```python
from build123d import *

# Parameters (mm, degrees)
BOSS_EXTRUDE1_DEPTH = 13.5
SKETCH2_W           = 45
SKETCH2_H           = 45
CUT_EXTRUDE1_DEPTH  = 11.72
SKETCH3_R           = 13.5
CUT_EXTRUDE2_DEPTH  = 84.329160712
CHAMFER1_SIZE       = 3
SKETCH7_W           = 113.25
SKETCH7_H           = 1.5
CUT_EXTRUDE4_DEPTH  = 84.598089841
CHAMFER2_SIZE       = 3
CHAMFER2_SIZE2      = 5.196152423
SKETCH8_R           = 2.25
CUT_EXTRUDE5_DEPTH  = 82.936336555
CUT_EXTRUDE6_START  = -4
SKETCH9_R           = 4.5
CUT_EXTRUDE6_DEPTH  = 78.936336555
SKETCH5_R           = 1.75
CUT_EXTRUDE7_DEPTH  = 84.013934059


with BuildPart() as part:
    # Sketch1 → Boss-Extrude1 (new body)
    with BuildSketch(Plane(origin=(0, 0, 0), x_dir=(1, 0, 0), z_dir=(0, 1, 0))):
        Polygon((-56.625, 0), (56.625, 0), (21.983983849, 60), (-21.983983849, 60), align=None)
    extrude(amount=BOSS_EXTRUDE1_DEPTH)

    # Sketch2 → Cut-Extrude1 (cut)
    with BuildSketch(Plane.XZ):
        with Locations((0, -31.45)):
            Rectangle(SKETCH2_W, SKETCH2_H)
    extrude(amount=-CUT_EXTRUDE1_DEPTH, mode=Mode.SUBTRACT)

    # Sketch3 → Cut-Extrude2 (cut, through all)
    with BuildSketch(Plane.XZ.offset(-11.72)):
        with Locations(Location((0, -31.45, 0), (0, 0, 270))):
            Circle(SKETCH3_R)
    extrude(amount=-CUT_EXTRUDE2_DEPTH, mode=Mode.SUBTRACT)

    # Chamfer1
    chamfer1_edges = [part.edges().sort_by_distance(p)[0] for p in [
        (-22.5, 5.86, -8.95),
        (-22.5, 5.86, -53.95),
        (22.5, 5.86, -53.95),
        (22.5, 5.86, -8.95),
    ]]
    chamfer(chamfer1_edges, length=CHAMFER1_SIZE)

    # Sketch7 → Cut-Extrude4 (cut, through all)
    with BuildSketch(Plane(origin=(0, 13.5, 0), x_dir=(1, 0, 0), z_dir=(0, 1, 0))):
        with Locations((0, 0.75)):
            Rectangle(SKETCH7_W, SKETCH7_H)
    extrude(amount=-CUT_EXTRUDE4_DEPTH, mode=Mode.SUBTRACT)

    # Chamfer2
    chamfer2_edges = [part.edges().sort_by_distance(p)[0] for p in [
        (0, 13.5, -1.5),
    ]]
    chamfer2_side = [part.faces().sort_by_distance(p)[0] for p in [
        (0, 6.75, -1.5),
    ]]
    chamfer(chamfer2_edges, length=CHAMFER2_SIZE, length2=CHAMFER2_SIZE2, reference=chamfer2_side[0])

    # Sketch8 → Cut-Extrude5 (cut, through all)
    with BuildSketch(Plane.XY.offset(-1.5)):
        with Locations((-40, 5)):
            Circle(SKETCH8_R)
        with Locations((40, 5)):
            Circle(SKETCH8_R)
    extrude(amount=-CUT_EXTRUDE5_DEPTH, mode=Mode.SUBTRACT)

    # Sketch9 → Cut-Extrude6 (cut, through all)
    with BuildSketch(Plane.XY.offset(-1.5).offset(CUT_EXTRUDE6_START)):
        with Locations((-40, 5)):
            Circle(SKETCH9_R)
        with Locations((40, 5)):
            Circle(SKETCH9_R)
    extrude(amount=-CUT_EXTRUDE6_DEPTH, mode=Mode.SUBTRACT)

    # Sketch5 → Cut-Extrude7 (cut, through all)
    with BuildSketch(Plane(origin=(0, 13.5, 0), x_dir=(1, 0, 0), z_dir=(0, 1, 0))):
        with Locations(Location((15.5, 46.95, 0), (0, 0, 270))):
            Circle(SKETCH5_R)
        with Locations(Location((15.5, 15.95, 0), (0, 0, 270))):
            Circle(SKETCH5_R)
        with Locations(Location((-15.5, 15.95, 0), (0, 0, 270))):
            Circle(SKETCH5_R)
        with Locations(Location((-15.5, 46.95, 0), (0, 0, 270))):
            Circle(SKETCH5_R)
    extrude(amount=-CUT_EXTRUDE7_DEPTH, mode=Mode.SUBTRACT)


solid = part.part
```
CAD build for the part. Positions are in the model's coordinates, mm. A direction names the side the tool comes from. Coordinates: 2 decimals unless noted, no trailing zeros. Order: outer loops, then holes, each group sorted by start corner. A loop starts at its lowest first (then second) coordinate and runs counter-clockwise, first axis right, second up.
(1) Which spindle directions (+Z, -Z, +X, -X, +Y, -Y) get a long thin tool onto all of the face, cutting with end or side? Do faces 4 (the face through (-38, 3, -5.5)), 5 (the face through (-20.98, 5.78, -10.43)), 6 (the face through (37.752, 5.099, -3.472)). Say none if no direction does.
Solution:
face 4: -Z
face 5: -Y
face 6: +Z, -Z
(2) Saw through at C-C, the plane z = -47.5. Write the cut outline in (x, y).
Solution:
outline: (-29.2, 0) - (-22.5, 0) - (-22.5, 11.72) - (-17.16, 11.72) - (-17.16, 13.5) - (-29.2, 13.5) - close; (-13.84, 11.72) - (13.84, 11.72) - (13.84, 13.5) - (-13.84, 13.5) - close; (17.16, 11.72) - (22.5, 11.72) - (22.5, 0) - (29.2, 0) - (29.2, 13.5) - (17.16, 13.5) - close
(3) Mould opens along X. For faces 1 (the face through (-0.8, 12, -4.1)), 2 (the face through (-38.635, 9.656, -31.159)), 3 (the face through (-20.98, 5.78, -52.47)) say: released by +X, released by -X, zero draft, split by the parting line, or undercut.
Solution:
face 1: zero draft
face 2: released by -X
face 3: undercut
(4) Saw through at A-A, the plane x = 15.5. Write the cut outline in (y, z).
Solution:
outline: (0, -60) - (13.5, -60) - (13.5, -48.7) - (11.72, -48.7) - (11.72, -53.95) - (0, -53.95) - close; (0, -8.95) - (11.72, -8.95) - (11.72, -14.2) - (13.5, -14.2) - (13.5, -6.7) - (10.5, -1.5) - (0, -1.5) - close; (11.72, -45.2) - (13.5, -45.2) - (13.5, -17.7) - (11.72, -17.7) - close
(5) Pin check, flat tips, straight feed: pin 1 Ø4 at (x, z) = (-15.5, -15.95) entering from +Y; pin 2 Ø2.5 at (x, y) = (41, 4) entering from -Z; pin 3 Ø2.5 at (x, y) = (-40, 5) entering from -Z; pin 4 Ø1 at (x, y) = (-28.5, 2) entering from -Z. Stop position of each tip, or through.
Solution:
pin 1: stops at y = 13.5
pin 2: stops at z = -5.5
pin 3: passes through
pin 4: stops at z = -49.58
(6) Saw through at B-B, the plane z = -19.5. Write the cut outline in (x, y), and give its area (3 significant figures).
Solution:
outline: (-45.37, 0) - (-22.5, 0) - (-22.5, 11.72) - (-6.28, 11.72) - (-6.28, 13.5) - (-45.37, 13.5) - close; (6.28, 11.72) - (22.5, 11.72) - (22.5, 0) - (45.37, 0) - (45.37, 13.5) - (6.28, 13.5) - close; hole circle Ø9 at (-40, 5); hole circle Ø9 at (40, 5)
area: 548 mm2
(7) Saw through at D-D, the plane x = -40. Write the cut outline in (y, z).
Solution:
outline: (0, -28.8) - (0.5, -28.8) - (0.5, -5.5) - (2.75, -5.5) - (2.75, -1.5) - (0, -1.5) - close; (7.25, -5.5) - (9.5, -5.5) - (9.5, -28.8) - (13.5, -28.8) - (13.5, -6.7) - (10.5, -1.5) - (7.25, -1.5) - close
(8) Drill centre lines: L1, parallel to Z at x = -5, y = 7.75; L2, parallel to Y at x = -40, z = -8; L3, parallel to X at y = 5, z = -25. Where is each one in solid material? Low to high.
Solution:
L1: z = -60 to -53.95, -8.95 to -1.5
L2: y = 0 to 0.5, 9.5 to 13.5
L3: x = -35.5 to -22.5, 22.5 to 35.5
